Model file for the job. Use its own axes, mm. Round coordinates to 2 decimals unless told otherwise and drop trailing zeros. Order: outer loops, then holes, each group sorted by start corner. A loop starts at its lowest first (then second) coordinate and runs counter-clockwise, first axis right, second up. Notation, with made-up numbers: (8.25, 44.25) - (63.25, 44.25) arc R16 cw to (63.25, 57.25) - close; hole circle Ø3 at (64.25, 44.5). An arc over 180 degrees is marked (long way). Use one line per item in the form item = value.
Autodesk Inventor part; units mm, degrees
ref_plane "YZ Plane" through (0, 0, 0) normal (1, 0, 0) x (0, 1, 0)
ref_plane "XZ Plane" through (0, 0, 0) normal (0, 1, 0) x (-1, 0, 0)
ref_plane "XY Plane" through (0, 0, 0) normal (0, 0, 1) x (1, 0, 0)
sketch "スケッチ1" plane through (0, 0, 0) normal (0, 0, 1) x (1, 0, 0)
  line L0 (25, 11) -> (-25, 11)
  line L1 (-25, 11) -> (-25, -11)
  line L2 (-25, -11) -> (25, -11)
  line L3 (25, -11) -> (25, 11)
  line L4 (25, 11) -> (-25, -11) construction
  line L5 (-25, 11) -> (25, -11) construction
  circle A0 centre (-20, 6) radius 1.6
  circle A1 centre (-20, -6) radius 1.6
  circle A2 centre (20, 6) radius 1.6
  circle A3 centre (20, -6) radius 1.6
  point P0 (0, 0)
  dimension "d0" = 50
  dimension "d1" = 22
  dimension "d14" = 3.2
  dimension "d15" = 3.2
  dimension "d16" = 3.2
  dimension "d17" = 3.2
  dimension "d18" = 40
  dimension "d19" = 5
  dimension "d20" = 12
  dimension "d21" = 5
extrude "押し出し1" add sketch "スケッチ1" along normal blind 8
sketch "スケッチ2" plane through (0, 0, 8) normal (0, 0, 1) x (1, 0, 0)
  circle A0 centre (0, 0) radius 5
  dimension "d4" = 10
hole "穴1" at (0, 0, 8) direction (0, 0, -1) diameter 8.647 end through all
fillet "フィレット1" radius 5 4 edges at (25, 11, 4) (25, -11, 4) (-25, 11, 4) (-25, -11, 4)
(1) Slice it at C-C on y = 0.75. Give the cut face in (x, z).
Report:
outline = (-25, 0) - (-4.26, 0) - (-4.26, 8) - (-25, 8) - close; (4.26, 0) - (25, 0) - (25, 8) - (4.26, 8) - close
(2) Pull direction Y, two halves, no side cores. Call faces 1 (the face through (18.73, -5.03, 3.94)), 2 (the face through (0, 11, 4)), 3 (the face through (25, 0, 4)): released by +Y, released by -Y, zero draft, split by the parting line, or undercut.
Report:
face_1 = undercut
face_2 = released by +Y
face_3 = zero draft
(3) Probe probe 1 along Y at (x, z) = (-20, 5.75); probe 2 along X at (y, z) = (0, 5); probe 3 along X at (y, z) = (-6.25, 4.25). List the from-to ranges inside material, lowest first. Write a range as [from, to].
Report:
probe_1 = [-11, -7.6], [-4.4, 4.4], [7.6, 11]
probe_2 = [-25, -4.32], [4.32, 25]
probe_3 = [-24.99, -21.58], [-18.42, 18.42], [21.58, 24.99]
(4) Slice it at B-B on x = 20.5. Give the cut face in (y, z), then the cut area to 3 significant figures.
Report:
outline = (-10.97, 0) - (-7.52, 0) - (-7.52, 8) - (-10.97, 8) - close; (-4.48, 0) - (4.48, 0) - (4.48, 8) - (-4.48, 8) - close; (7.52, 0) - (10.97, 0) - (10.97, 8) - (7.52, 8) - close
area = 127 mm2
(5) Slice it at D-D on y = -3.25. Give the cut face in (x, z).
Report:
outline = (-25, 0) - (-2.85, 0) - (-2.85, 8) - (-25, 8) - close; (2.85, 0) - (25, 0) - (25, 8) - (2.85, 8) - close
(6) Slice it at A-A on z = 6. Give the cut face in (x, y), then the cut area to 3 significant figures.
Report:
outline = (-25, -6) arc R5 ccw to (-20, -11) - (20, -11) arc R5 ccw to (25, -6) - (25, 6) arc R5 ccw to (20, 11) - (-20, 11) arc R5 ccw to (-25, 6) - close; hole circle Ø3.2 at (-20, -6); hole circle Ø3.2 at (-20, 6); hole circle Ø8.65 at (0, 0); hole circle Ø3.2 at (20, -6); hole circle Ø3.2 at (20, 6)
area = 988 mm2
